Autodesk Inventor part; units mm, degrees
ref_plane "YZ Plane" through (0, 0, 0) normal (1, 0, 0) x (0, 1, 0)
ref_plane "XZ Plane" through (0, 0, 0) normal (0, 1, 0) x (-1, 0, 0)
ref_plane "XY Plane" through (0, 0, 0) normal (0, 0, 1) x (1, 0, 0)
sketch "Sketch1" plane through (0, 0, 0) normal (0, 0, 1) x (1, 0, 0)
  line L0 (381.5852, -185.7682) -> (94.217, 105.9508)
  line L1 (94.217, 105.9508) -> (-70.883, 105.9508)
  line L2 (-70.883, 105.9508) -> (-358.2512, -185.7682)
  line L3 (1105.6551, 353.06) -> (-810.8916, 353.06) construction
  line L4 (381.5852, -185.7682) -> (-358.2512, -185.7682)
  dimension "d4" = 165.1
  dimension "d7" = 291.719
extrude "Plate1" add sketch "Sketch1" along normal blind 3.048
sketch "Sketch2" plane through (0, 0, 3.048) normal (0, 0, 1) x (1, 0, 0)
  line L0 (94.217, 105.9508) -> (381.5852, -185.7682) construction
  line L1 (-70.883, 105.9508) -> (94.217, 105.9508) construction
  line L2 (-358.2512, -185.7682) -> (-70.883, 105.9508) construction
  line L3 (381.5852, -185.7682) -> (-358.2512, -185.7682) construction
  line L4 (11.667, 105.9508) -> (11.667, -185.7682) construction
  point P0 (0, 0)
  point P1 (24.367, 64.6758)
  point P2 (24.367, 39.2758)
  point P3 (-1.033, 64.6758)
  point P4 (-1.033, 39.2758)
  dimension "d8" = 12.7
  dimension "d9" = 41.275
  dimension "d10" = 25.4
hole "Hole1" at (24.367, 64.6758, 3.048) at (24.367, 39.2758, 3.048) at (-1.033, 39.2758, 3.048) at (-1.033, 64.6758, 3.048) direction (0, 0, -1) diameter 5.1054 end through all
sketch "Sketch3" plane through (0, 0, 0) normal (0, 0, -1) x (-1, 0, 0)
  circle A0 centre (1.033, 64.6758) radius 2.5527 construction
  circle A1 centre (1.033, 39.2758) radius 2.5527 construction
  circle A2 centre (-24.367, 39.2758) radius 2.5527 construction
  circle A3 centre (-24.367, 64.6758) radius 2.5527 construction
  line L0 (-94.217, 105.9508) -> (70.883, 105.9508)
  line L1 (-381.5852, -185.7682) -> (-94.217, 105.9508) construction
  line L2 (358.2512, -185.7682) -> (-381.5852, -185.7682) construction
  line L3 (70.883, 105.9508) -> (358.2512, -185.7682) construction
  line L4 (115.4456, 60.7134) -> (110.9219, 56.2572)
  line L5 (110.9219, 56.2572) -> (66.3592, 101.4945)
  line L6 (66.3592, 101.4945) -> (70.883, 105.9508)
  line L7 (70.883, 105.9508) -> (115.4456, 60.7134)
  line L8 (66.3592, 101.4945) -> (61.9694, 105.9508)
  line L9 (-11.667, 105.9508) -> (-11.667, 80.5508) construction
  line L10 (-11.667, 105.9508) -> (13.733, 105.9508) construction
  line L11 (-138.7797, 60.7134) -> (-134.256, 56.2572)
  line L12 (-134.256, 56.2572) -> (-89.6933, 101.4945)
  line L13 (-94.217, 105.9508) -> (-138.7797, 60.7134)
  line L14 (-89.6933, 101.4945) -> (-85.3035, 105.9508)
  line L15 (-85.3035, 105.9508) -> (-134.256, 56.2572)
  line L16 (-134.256, 56.2572) -> (-138.7797, 60.7134)
  line L17 (-138.7797, 60.7134) -> (-94.217, 105.9508)
  line L18 (-94.217, 105.9508) -> (-85.3035, 105.9508)
  line L19 (70.883, 105.9508) -> (61.9694, 105.9508)
  point P0 (0, 0)
  dimension "d18" = 6.35
  dimension "d19" = 63.5
  dimension "d20" = 25.4
  dimension "d21" = 90
extrude "Cut1" cut sketch "Sketch3" against normal blind 3.048
fillet "Corner Round1" radius 6.35 2 edges at (-358.2512, -185.7682, 1.524) (381.5852, -185.7682, 1.524)
fillet "Corner Round2" radius 127 2 edges at (-110.9219, 56.2572, 1.524) (134.256, 56.2572, 1.524)
equation "\"d16\" = Thickness"
equation "\"d22\" = Thickness"
equation "\"d2\" = Thickness"
equation "\"BendRadius\" = Thickness"
equation "\"BendReliefWidth\" = Thickness"
equation "\"BendReliefDepth\" = 0.5 * Thickness"
equation "\"CornerReliefSize\" = 4 * Thickness"
equation "\"MinimumRemnant\" = 2 * Thickness"
equation "\"TransitionRadius\" = BendRadius"
equation "\"JacobiRadiusSize\" = BendRadius"
equation "\"GapSize\" = Thickness"
properties part number "hopper_back_plate" material "Polycarbonate, Smoke"
Can you work these out from the model? Positions are in its coordinate system, mm. Give positions to 0.01 mm unless a question says otherwise; leave off trailing zeros. Loops run counter-clockwise (first coordinate to the right, second up) from the corner with the lowest first, then second, coordinate; pieces in that order, holes last. Notation, with made-up numbers: M 81.5,81.5 L 85.5,81.5 A11 ccw 85.5,101.5 Z; hole C -12,-22 d10. An arc over 180 degrees is marked long. One line per item, written item: value. Start each with the question number.
1) Thinking about a two-plate mould opening in X: for faces 1 (the face through (256.485, -58.774, 1.503)), 2 (the face through (-229.901, -55.475, 1.503)), 3 (the face through (7, -70, 0)), which applies, +X half, -X half, draft (parallel to the pull), parting line (faces both ways), or undercut?
2) If I drill on line 1 (X direction, y = 67, z = 0.4); line 2 (Y direction, x = 195, z = 1.4); line 3 (X direction, y = 15, z = 1.9), over which ranges is the centre line in solid material (lowest first)? Write a range as [from, to].
3) If we section it at B-B, the plane y = -39: Write out the boundary of the cut face in (x, z).
4) If we section it at A-A, the plane z = 2.45: Write out the boundary of the cut face in (x, y), and give its area (3 significant figures).
5) I'm going to push a flat-ended pin straight in: pin 1 (1 mm diameter, centred on y = -19, z = 2, fed in from +X). Where does the tip first touch, or does it pass through?
6) If we section it at C-C, the plane x = 115.5: Write out the boundary of the cut face in (y, z), and give its area (3 significant figures).
Completed:
1. face 1: +X half
1. face 2: -X half
1. face 3: draft
2. line 1: x = [-104.59, -2.09], [0.02, 23.31], [25.42, 127.92]
2. line 2: y = [-185.77, 3.64]
2. line 3: x = [-160.48, 183.81]
3. outline: M -213.67,0 L 237.01,0 L 237.01,3.05 L -213.67,3.05 Z
4. outline: M -347.61,-174.96 A6.35 ccw -343.08,-185.77 L 366.42,-185.77 A6.35 ccw 370.94,-174.96 L 138.78,60.71 A127 cw 106.43,84.51 L 89.69,101.49 L 85.3,105.95 L -61.97,105.95 L -66.36,101.49 L -83.09,84.51 A127 cw -115.45,60.71 Z; hole C -1.03,39.28 d5.11; hole C -1.03,64.68 d5.11; hole C 24.37,39.28 d5.11; hole C 24.37,64.68 d5.11
4. area: 131,000 mm^2
5. pin 1: stops at x = 217.8
6. outline: M -185.77,0 L 76.15,0 L 76.15,3.05 L -185.77,3.05 Z
6. area: 798 mm^2
